Check sheet for the drawn part. Datum: minimum x, y, z corner. Units: mm. Coordinates: 2 decimals unless noted, no trailing zeros. Write each loop counter-clockwise with the first axis right and the second up, starting at its lowest first coordinate (ties: lowest second). Pieces come first, ordered by that corner, then holes. Notation, with made-up numbers: (61.25, 49) - (111.25, 49) arc R30 ccw to (111.25, 78) - close; hole circle Ø5 at (48.25, -22). An arc over 180 degrees is marked (long way). Write each question's results on one line, items separated by ' | '.
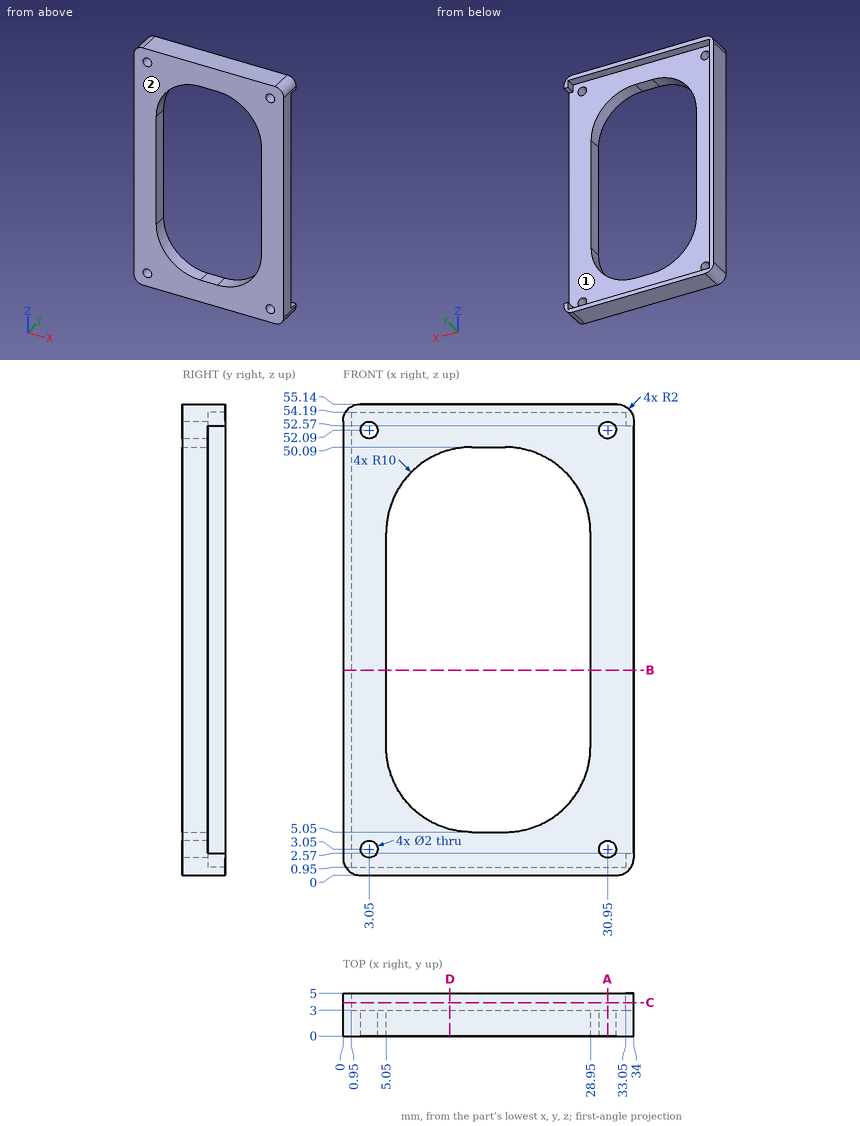
1. Sectioned sample at B-B (z = 24). Record the cut outline in (x, y), then the cut area to 3 significant figures.
Values follow:
outline: (0, 0) - (5.05, 0) - (5.05, 3) - (0.95, 3) - (0.95, 5) - (0, 5) - close; (28.95, 0) - (34, 0) - (34, 3) - (28.95, 3) - close | area: 32.2 mm^2
2. Go/stop test with flat-tipped pins: pin 1 (1 mm diameter, centred on y = 4, z = 33.5, fed in from +X); pin 2 (8 mm diameter, centred on x = 23.5, z = 16.5, fed in from -Y); pin 3 (3 mm diameter, centred on x = 3.05, z = 52.09, fed in from +Y); pin 4 (3 mm diameter, centred on y = 1.5, z = 22.5, fed in from -X). Record where each tip stops, or that it passes through.
Values follow:
pin 1: stops at x = 0.95 | pin 2: passes through | pin 3: stops at y = 3 | pin 4: stops at x = 0
3. Draft check along Z on the marked faces 1 and 2. Enter one of: pulls with the +Z half, pulls with the -Z half, needs draft (parallel to the pull), parting line crosses it, or undercut.
Values follow:
face 1: undercut | face 2: needs draft
4. Material ranges on L1, parallel to X at y = 1.5, z = 52.09; L2, parallel to X at y = 1.9, z = 35; L3, parallel to Z at x = 19.5, y = 3.8, recorded low to high. Write a range as [from, to].
Values follow:
L1: x = [0, 2.05], [4.05, 29.95], [31.95, 34] | L2: x = [0, 5.05], [28.95, 34] | L3: z = [0, 0.95], [54.19, 55.14]
5. Sectioned sample at D-D (x = 12.5). Record the cut outline in (y, z).
Values follow:
outline: (0, 0) - (5, 0) - (5, 0.95) - (3, 0.95) - (3, 5.38) - (0, 5.38) - close; (0, 49.76) - (3, 49.76) - (3, 54.19) - (5, 54.19) - (5, 55.14) - (0, 55.14) - close
6. Sectioned sample at A-A (x = 30.95). Record the cut outline in (y, z).
Values follow:
outline: (0, 0) - (5, 0) - (5, 0.95) - (3, 0.95) - (3, 2.05) - (0, 2.05) - close; (0, 4.05) - (3, 4.05) - (3, 51.09) - (0, 51.09) - close; (0, 53.09) - (3, 53.09) - (3, 54.19) - (5, 54.19) - (5, 55.14) - (0, 55.14) - close
7. Sectioned sample at C-C (y = 3.9). Record the cut outline in (x, z).
Values follow:
outline: (0, 2) arc R2 ccw to (2, 0) - (32, 0) arc R2 ccw to (34, 2) - (34, 2.57) - (33.05, 2.57) - (33.05, 0.95) - (0.95, 0.95) - (0.95, 54.19) - (33.05, 54.19) - (33.05, 52.57) - (34, 52.57) - (34, 53.14) arc R2 ccw to (32, 55.14) - (2, 55.14) arc R2 ccw to (0, 53.14) - close
